The listing builds one solid part. Answer for the finished solid, in the listing's coordinates (mm). Face numbers are marked on the shaded views. A direction names the side the tool comes from. Round coordinates to 2 decimals unless told otherwise and drop trailing zeros. Loops run counter-clockwise (first coordinate to the right, second up) from the corner with the lowest first, then second, coordinate; pieces in that order, holes last. Notation, with made-up numbers: (49.5, 19) - (70.5, 19) arc R10 ccw to (70.5, 38) - close; hole circle Ø4 at (32.5, 30.25). An arc over 180 degrees is marked (long way). One line per item, written item: value.
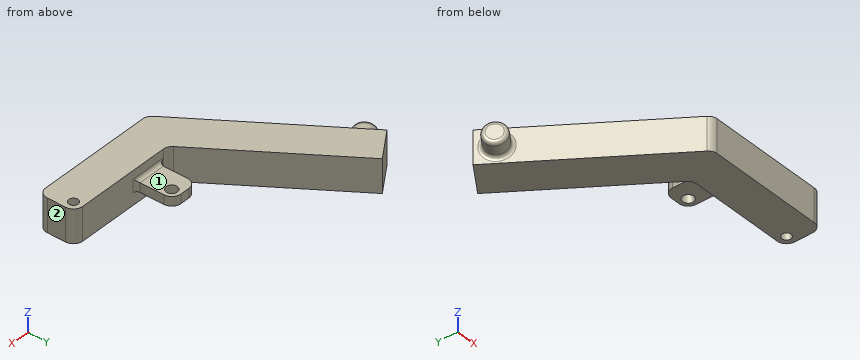
Autodesk Inventor part; units mm, degrees
ref_plane "YZ Plane" through (0, 0, 0) normal (1, 0, 0) x (0, 1, 0)
ref_plane "XZ Plane" through (0, 0, 0) normal (0, 1, 0) x (-1, 0, 0)
ref_plane "XY Plane" through (0, 0, 0) normal (0, 0, 1) x (1, 0, 0)
sketch "Sketch1" plane through (0, 0, 0) normal (0, 0, 1) x (1, 0, 0)
  line L0 (0, 0) -> (-59.4775, 0)
  line L1 (0, 0) -> (0, -20)
  line L2 (0, -20) -> (-70, -20)
  circle A0 centre (-5, -5) radius 2.5
  line L3 (-59.4775, 0) -> (-110.1581, 73.7407)
  line L4 (-110.1581, 73.7407) -> (-126.6406, 62.4126)
  line L5 (-126.6406, 62.4126) -> (-70, -20)
  line L6 (-5, -5) -> (93.9651, 63.0168)
  line L7 (-5, -5) -> (-119.3081, 161.3193)
  dimension "d1" = 5
  dimension "d2" = 20
  dimension "d3" = 5
  dimension "d4" = 5
  dimension "d50" = 70
  dimension "d51" = 124.5
  dimension "d52" = 20
  dimension "d53" = 100
  dimension "d55" = 34.5
extrude "Extrusion1" add sketch "Sketch1" along normal blind 18 contours L1 L6 A0 L7 L0 | L7 A0 L6 L1 L2 L5 L4 L3 L0
fillet "Fillet5" radius 5 2 edges at (0, 0, 9) (0, -20, 9)
sketch "Sketch5" plane through (-70, 0, 0) normal (0, 1, 0) x (1, 0, 0)
  line L0 (15.5225, 0) -> (30.5225, 0)
  line L1 (30.5225, 0) -> (30.5225, -11.5)
  line L2 (30.5225, -11.5) -> (15.5225, -11.5)
  line L3 (15.5225, -11.5) -> (15.5225, 0)
  line L4 (65, -18) -> (10.5225, -18)
  line L5 (0, 0) -> (0, -18)
  line L6 (65, 0) -> (10.5225, 0)
  line L7 (10.5225, 0) -> (10.5225, -18)
  point P0 (70, 0)
  point P1 (0, -3.5)
  dimension "d31" = 15
  dimension "d33" = 6.5
  dimension "d54" = 20
extrude "Extrusion5" add sketch "Sketch5" along normal blind 20
sketch "Sketch6" plane through (-39.4775, 0, 11.5) normal (0, 0, 1) x (1, 0, 0)
  circle A0 centre (-5, 15) radius 3
  line L0 (-15, 20) -> (0, 20)
  line L1 (0, 0) -> (0, 20)
  point P0 (39.4775, 0)
  dimension "d37" = 6
  dimension "d38" = 5
  dimension "d39" = 5
extrude "Extrusion6" cut sketch "Sketch6" against normal up to next
sketch "Sketch7" plane through (-54.4775, 0, 0) normal (-1, 0, 0) x (0, 0, 1)
  line L0 (0, 20) -> (6.5, 20)
  line L1 (0, 0) -> (0, 20)
  line L2 (6.5, 20) -> (6.5, 0)
  line L3 (6.5, 0) -> (0, 0)
  line L4 (0, 0) -> (0, 20)
  line L5 (11.5, 0) -> (11.5, 20)
  line L6 (0, 20) -> (11.5, 20)
  dimension "d42" = 5
  dimension "d44" = 20
extrude "Extrusion7" cut sketch "Sketch7" against normal up to next
fillet "Fillet8" radius 5 2 edges at (-39.4775, 20, 9) (-54.4775, 20, 9)
fillet "Fillet9" radius 2 3 edges at (-54.4775, 0, 9) (-46.9775, 0, 11.5) (-39.4775, 0, 9)
sketch "Sketch8" plane through (-70, -20, 0) normal (-0.8241, -0.5664, 0) x (0, 0, 1)
  circle A0 centre (9, 90) radius 6
  line L0 (0, 100) -> (18, 100)
  line L1 (18, 100) -> (18, 0)
  point P0 (0, -23.1659)
  dimension "d56" = 12
  dimension "d57" = 10
  dimension "d58" = 9
extrude "Extrusion8" add sketch "Sketch8" along normal blind 10
fillet "Fillet11" radius 2 2 edges at (-129.2178, 48.5073, 3) (-120.9766, 54.1714, 3)
fillet "Fillet12" radius 5 2 edges at (-70, -20, 9) (-59.4775, 0, 9)
properties part number "Swinging_connection" material "Wood (Cherry)"
1) Consider L1, parallel to Y at x = -5, z = 6; L2, parallel to Y at x = -36.5, z = 11.75; L3, parallel to X at y = -4, z = 11. Determine where each line is inside the solid, lowest interval first.
Final values:
L1: -20 to -7.5, -2.5 to 0
L2: -20 to 0
L3: -81 to -7.29, -2.71 to -0.1
2) For the marked faces 1 and 2, determine the directions among +Z, -Z, +X, -X, +Y, -Y from which every point of the face is accessible in a straight line to the end or side of a thin tool.
Final values:
face 1: +Z, +X, +Y
face 2: +Z, -Z, +X, +Y, -Y
3) Each of these flat-tipped pins is pushed along its axis until it touches: pin 1 Ø8 at (y, z) = (9.5, 15) entering from +X; pin 2 Ø5 at (y, z) = (56.5, 7) entering from -X; pin 3 Ø1.5 at (x, z) = (-48, 9.5) entering from +Y; pin 4 Ø10 at (x, y) = (-118, 48.5) entering from +Z. Where does it stop, or does it pass through?
Final values:
pin 1: x = -39.48
pin 2: x = -131.29
pin 3: y = 20
pin 4: z = 18
4) A cutting plane is placed at A-A on x = -21.5. Give the vertices of the cut face in (y, z).
Final values:
outline: (-20, 0) - (0, 0) - (0, 18) - (-20, 18) - close
5) A cutting plane is placed at B-B on y = 29.5. Give the vertices of the cut face in (x, z).
Final values:
outline: (-104.02, 0) - (-79.75, 0) - (-79.75, 18) - (-104.02, 18) - close
